from build123d import *

# Parameters (mm, degrees)
F0_W     = 100
F0_H     = 40
F1_DEPTH = 30
F2_W     = 15
F2_H     = 10
F3_DEPTH = 10


with BuildPart() as f1:
    # F0 (on Top) → F1 (new body, symmetric)
    with BuildSketch(Plane.XY):
        with Locations((-50, 20)):
            Rectangle(F0_W, F0_H)
    extrude(amount=F1_DEPTH, both=True)

    # F2 (on face) → F3 (join)
    with BuildSketch(Plane.XY.offset(30)):
        with Locations((-7.5, 20)):
            Rectangle(F2_W, F2_H)
    extrude(amount=F3_DEPTH)


solid = f1.part
Here's how the part is built. I have some questions about the finished solid (model axes, mm). A direction names the side the tool comes from. Coordinates: 2 decimals unless noted, no trailing zeros. Loops run counter-clockwise (first coordinate to the right, second up) from the corner with the lowest first, then second, coordinate; pieces in that order, holes last.
1. Imagine slicing it at C-C, the plane x = -90. Please give me the cut outline in (y, z), and give its area (3 significant figures).
2. For P1, Ø6, axis at y = 18, z = -19.5, coming from the +X side; P2, Ø4, axis at x = -14.5, z = 33, coming from the +Y side; P3, Ø8, axis at x = -80, y = 9.5, coming from the +Z side; P4, Ø8, axis at y = 20.5, z = 36, coming from the -X side, each with a flat end and sliding along its axis, tell me the tip position at first contact or that it passes through.
3. Imagine slicing it at A-A, the plane x = -10. Please give me the cut outline in (y, z), and give its area (3 significant figures).
4. Imagine slicing it at B-B, the plane y = 21. Please give me the cut outline in (x, z), and give its area (3 significant figures).
5. Imagine slicing it at D-D, the plane y = 11. Please give me the cut outline in (x, z), and give its area (3 significant figures).
6. I need wall thicknesses on L1, parallel to Z at x = -67, y = 7; L2, parallel to Y at x = -7.5, z = 33. Which ranges of each line are inside material? Lowest first, please.
7. For faces 1 (the flat face through (-8, 15, 35)), 2 (the flat face through (-15, 20, 35)), 3 (the flat face through (-8, 25, 35)), which set-ups out of +Z, -Z, +X, -X, +Y, -Y let a thin tool reach every point of the face, with its end or its side?
Taken from the geometry:
1. outline: (0, -30) - (40, -30) - (40, 30) - (0, 30) - close
1. area: 2,400 mm2
2. P1: stops at x = 0
2. P2: stops at y = 25
2. P3: stops at z = 30
2. P4: stops at x = -15
3. outline: (0, -30) - (40, -30) - (40, 30) - (25, 30) - (25, 40) - (15, 40) - (15, 30) - (0, 30) - close
3. area: 2,500 mm2
4. outline: (-100, -30) - (0, -30) - (0, 40) - (-15, 40) - (-15, 30) - (-100, 30) - close
4. area: 6,150 mm2
5. outline: (-100, -30) - (0, -30) - (0, 30) - (-100, 30) - close
5. area: 6,000 mm2
6. L1: z = -30 to 30
6. L2: y = 15 to 25
7. face 1: +Z, +X, -X, -Y
7. face 2: +Z, -X, +Y, -Y
7. face 3: +Z, +X, -X, +Y
